Geometry: final body of the model. Coordinates: model frame, mm. Give positions to 0.01 mm unless a question says otherwise; leave off trailing zeros. Loops run counter-clockwise (first coordinate to the right, second up) from the corner with the lowest first, then second, coordinate; pieces in that order, holes last.
from build123d import *

# Parameters (mm, degrees)
BOSS_EXTRUDE1_DEPTH = 2
CUT_EXTRUDE1_DEPTH  = 2


with BuildPart() as part:
    # Sketch1 → Boss-Extrude1 (new body)
    with BuildSketch(Plane.XY):
        with BuildLine():
            Line((10, 0), (240, 0))
            ThreePointArc((240, 0), (247.071067812, 2.928932188), (250, 10))
            Line((250, 10), (250, 240))
            ThreePointArc((250, 240), (247.071067812, 247.071067812), (240, 250))
            Line((240, 250), (10, 250))
            ThreePointArc((10, 250), (2.928932188, 247.071067812), (0, 240))
            Line((0, 240), (0, 160))
            ThreePointArc((0, 160), (-2.928932188, 152.928932188), (-10, 150))
            Line((-10, 150), (-110, 150))
            ThreePointArc((-110, 150), (-117.071067812, 147.071067812), (-120, 140))
            Line((-120, 140), (-120, 110))
            ThreePointArc((-120, 110), (-117.071067812, 102.928932188), (-110, 100))
            Line((-110, 100), (-10, 100))
            ThreePointArc((-10, 100), (-2.928932188, 97.071067812), (0, 90))
            Line((0, 90), (0, 10))
            ThreePointArc((0, 10), (2.928932188, 2.928932188), (10, 0))
        make_face()
    extrude(amount=BOSS_EXTRUDE1_DEPTH)

    # Sketch2 → Cut-Extrude1 (cut)
    with BuildSketch(Plane.XY.offset(2)):
        with BuildLine():
            Line((121.831245853, 74.238883319), (81.553468075, 158.375168042))
            Line((81.553468075, 158.375168042), (81.553468075, 92.294438875))
            add(Edge.make_bspline(
                [(81.553468075, 92.294438875), (81.552441695, 91.527408259), (81.550494213, 90.07202371), (81.67476659, 88.003330285), (81.809557178, 86.154926562), (82.033410561, 84.535090304), (82.270961447, 83.126350994), (82.624899995, 81.963045824), (82.992758599, 80.996359886), (83.345604613, 80.48395593), (83.506593075, 80.250168042)],
                knots=[0, 0, 0, 0, 1.48973486, 2.826663046, 4.025252461, 5.088590954, 6.003687083, 6.795186099, 7.45029523, 8, 8, 8, 8], degree=3))
            add(Edge.make_bspline(
                [(83.506593075, 80.250168042), (83.997407371, 79.750770196), (84.996905643, 78.733792313), (87.003759394, 77.711270113), (89.366130367, 77.105906039), (91.068976257, 77.047545775), (91.970134742, 77.016661097)],
                knots=[0, 0, 0, 0, 0.893460505, 1.819450328, 2.846037184, 4, 4, 4, 4], degree=3))
            Line((91.970134742, 77.016661097), (95.442356964, 77.016661097))
            Line((95.442356964, 77.016661097), (95.442356964, 74.238883319))
            Line((95.442356964, 74.238883319), (60.720134742, 74.238883319))
            Line((60.720134742, 74.238883319), (60.720134742, 77.016661097))
            Line((60.720134742, 77.016661097), (64.192356964, 77.016661097))
            add(Edge.make_bspline(
                [(64.192356964, 77.016661097), (64.692336968, 77.027575423), (65.660187495, 77.048703141), (67.053155801, 77.255679207), (68.340072371, 77.542980734), (69.511077493, 77.990029314), (70.577284489, 78.54537262), (71.523997685, 79.246760067), (72.334604766, 80.088398233), (72.793088669, 80.714808629), (73.024822242, 81.031418042)],
                knots=[0, 0, 0, 0, 1.182386838, 2.288838982, 3.326958154, 4.296765023, 5.246416275, 6.164047556, 7.072046332, 8, 8, 8, 8], degree=3))
            add(Edge.make_bspline(
                [(73.024822242, 81.031418042), (73.154175481, 81.267158908), (73.438935547, 81.786122213), (73.754068555, 82.7087764), (73.999815936, 83.832477906), (74.243351558, 85.140425739), (74.413930293, 86.655788373), (74.502709761, 88.358707772), (74.607417007, 90.260571867), (74.608469203, 91.592574666), (74.609023631, 92.294438875)],
                knots=[0, 0, 0, 0, 0.561580455, 1.236271222, 2.028879402, 2.966584022, 4.017422664, 5.2149421, 6.532486222, 8, 8, 8, 8], degree=3))
            Line((74.609023631, 92.294438875), (74.609023631, 156.183327764))
            add(Edge.make_bspline(
                [(74.609023631, 156.183327764), (74.598097419, 157.262279808), (74.57781297, 159.265348068), (74.292147678, 162.020464101), (73.887395445, 164.316152629), (73.38248359, 165.621386735), (73.155030575, 166.20936943)],
                knots=[0, 0, 0, 0, 1.269100049, 2.356076937, 3.259444487, 4, 4, 4, 4], degree=3))
            add(Edge.make_bspline(
                [(73.155030575, 166.20936943), (72.964440038, 166.571330676), (72.572351095, 167.315968917), (71.739346077, 168.310495354), (70.678433406, 169.192456789), (69.404596857, 170.014029453), (67.793926343, 170.70426646), (65.790057774, 171.151821363), (63.389943364, 171.426827209), (61.654210729, 171.449112709), (60.720134742, 171.461105542)],
                knots=[0, 0, 0, 0, 0.685675889, 1.410594349, 2.160436148, 2.996293973, 3.94870651, 5.086176952, 6.431940446, 8, 8, 8, 8], degree=3))
            Line((60.720134742, 171.461105542), (60.720134742, 174.238883319))
            Line((60.720134742, 174.238883319), (89.192356964, 174.238883319))
            Line((89.192356964, 174.238883319), (126.38853752, 96.547911097))
            Line((126.38853752, 96.547911097), (163.584718075, 174.238883319))
            Line((163.584718075, 174.238883319), (191.275690297, 174.238883319))
            Line((191.275690297, 174.238883319), (191.275690297, 171.461105542))
            Line((191.275690297, 171.461105542), (187.868572242, 171.461105542))
            add(Edge.make_bspline(
                [(187.868572242, 171.461105542), (187.361287545, 171.450707073), (186.386065744, 171.430716694), (184.979607429, 171.218940655), (183.683652592, 170.938748781), (182.506844601, 170.48708074), (181.439074078, 169.933617837), (180.493564629, 169.223853404), (179.660586682, 168.397082941), (179.201520738, 167.764165368), (178.971002797, 167.446348597)],
                knots=[0, 0, 0, 0, 1.192663738, 2.292818382, 3.341598875, 4.305885976, 5.250132179, 6.162540657, 7.077327887, 8, 8, 8, 8], degree=3))
            add(Edge.make_bspline(
                [(178.971002797, 167.446348597), (178.841649558, 167.210607731), (178.556889492, 166.691644426), (178.241756484, 165.768990238), (177.996009103, 164.645288733), (177.752473481, 163.3373409), (177.581894746, 161.821978266), (177.493115279, 160.119058867), (177.388408032, 158.217194771), (177.387355836, 156.885191972), (177.386801408, 156.183327764)],
                knots=[0, 0, 0, 0, 0.561580455, 1.236271222, 2.028879402, 2.966584022, 4.017422664, 5.2149421, 6.532486222, 8, 8, 8, 8], degree=3))
            Line((177.386801408, 156.183327764), (177.386801408, 92.294438875))
            add(Edge.make_bspline(
                [(177.386801408, 92.294438875), (177.385877428, 91.527429602), (177.384124243, 90.072085551), (177.507098339, 88.003121526), (177.646069278, 86.155589108), (177.85710522, 84.531668283), (178.13424254, 83.12975452), (178.473014721, 81.957654643), (178.8699969, 80.994203331), (179.237061444, 80.483751398), (179.405030575, 80.250168042)],
                knots=[0, 0, 0, 0, 1.486776415, 2.821049613, 4.017258766, 5.078485589, 5.994452933, 6.784380121, 7.443731031, 8, 8, 8, 8], degree=3))
            add(Edge.make_bspline(
                [(179.405030575, 80.250168042), (179.895423699, 79.749880201), (180.898563608, 78.726499826), (182.913754693, 77.721375862), (185.270314869, 77.101877529), (186.966975459, 77.046231247), (187.868572242, 77.016661097)],
                knots=[0, 0, 0, 0, 0.893634595, 1.828003868, 2.845812335, 4, 4, 4, 4], degree=3))
            Line((187.868572242, 77.016661097), (191.275690297, 77.016661097))
            Line((191.275690297, 77.016661097), (191.275690297, 74.238883319))
            Line((191.275690297, 74.238883319), (149.609023631, 74.238883319))
            Line((149.609023631, 74.238883319), (149.609023631, 77.016661097))
            Line((149.609023631, 77.016661097), (153.081245853, 77.016661097))
            add(Edge.make_bspline(
                [(153.081245853, 77.016661097), (153.588433734, 77.027378344), (154.563469412, 77.047981553), (155.964240322, 77.254470656), (157.255601407, 77.548600741), (158.43409031, 77.978736677), (159.491525168, 78.55248399), (160.434038314, 79.246610187), (161.24579725, 80.082629427), (161.690291414, 80.714044665), (161.913711131, 81.031418042)],
                knots=[0, 0, 0, 0, 1.198333024, 2.303717216, 3.340834392, 4.325725627, 5.259386468, 6.176132048, 7.08325442, 8, 8, 8, 8], degree=3))
            add(Edge.make_bspline(
                [(161.913711131, 81.031418042), (162.04306437, 81.267158908), (162.327824436, 81.786122213), (162.642957444, 82.7087764), (162.888704825, 83.832477906), (163.132240447, 85.140425739), (163.302819182, 86.655788373), (163.391598649, 88.358707772), (163.496305896, 90.260571867), (163.497358092, 91.592574666), (163.49791252, 92.294438875)],
                knots=[0, 0, 0, 0, 0.561580455, 1.236271222, 2.028879402, 2.966584022, 4.017422664, 5.2149421, 6.532486222, 8, 8, 8, 8], degree=3))
            Line((163.49791252, 92.294438875), (163.49791252, 158.375168042))
            Line((163.49791252, 158.375168042), (123.220134742, 74.238883319))
            Line((123.220134742, 74.238883319), (121.831245853, 74.238883319))
        make_face()
    extrude(amount=-CUT_EXTRUDE1_DEPTH, mode=Mode.SUBTRACT)


solid = part.part
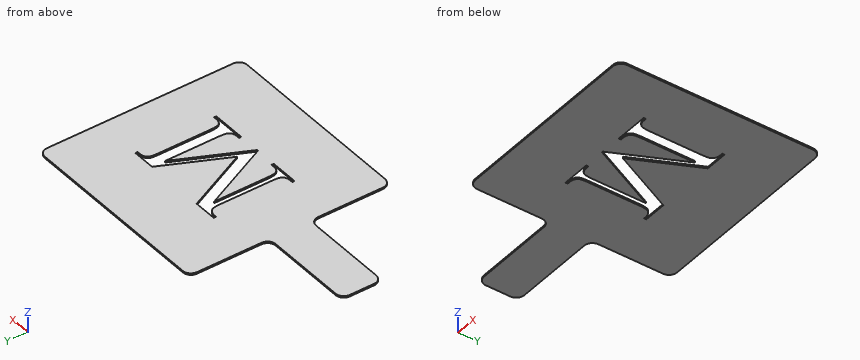
Item 1: Ray query, probe 1 along X at (y, z) = (133, 0.45); probe 2 along X at (y, z) = (87, 0.1); probe 3 along X at (y, z) = (162, 1.4). Return the intervals inside material, ascending.
Values follow:
probe 1: x = -120 to 74.61, 81.55 to 93.7, 108.94 to 143.84, 151.35 to 163.5, 177.39 to 250
probe 2: x = 0 to 74.42, 81.75 to 115.72, 129.33 to 163.31, 177.59 to 250
probe 3: x = 0 to 74.26, 95.05 to 157.73, 177.61 to 250
Item 2: Section query A-A on y = 181.5. Return loops of the section in (x, z).
Values follow:
outline: (0, 0) - (250, 0) - (250, 2) - (0, 2) - close
Item 3: Pin query (flat end, axial travel): pin 1 (0.6 mm diameter, centred on y = 75.5, z = 1.5, fed in from -X); pin 2 (0.6 mm diameter, centred on x = -58.5, z = 1, fed in from -Y); pin 3 (1 mm diameter, centred on x = -56, z = 0.5, fed in from +Y). Return the tip coordinate at first contact, or that it passes through.
Values follow:
pin 1: stops at x = 0
pin 2: stops at y = 100
pin 3: stops at y = 150
